Design review of the part built by this model. Coordinates are the model's own, in mm. A direction names the side the tool comes from. Round coordinates to 2 decimals unless told otherwise and drop trailing zeros. Order: outer loops, then holes, each group sorted by start corner. A loop starts at its lowest first (then second) coordinate and runs counter-clockwise, first axis right, second up. Notation, with made-up numbers: M 88,7.25 L 99,7.25 A34 cw 99,38.25 Z; hole C -32,-15 d7. An arc over 180 degrees is marked long. Write each question's results on one line, items separated by ' | '. Start each with the question number.
Item 1: Machinability: for faces 5 (the flat face through (-1, 50, 71)), 6 (the flat face through (150, 219, 573)), 7 (the flat face through (-4, 69, 140)), 8 (the flat face through (199, -150, 69)), which of the approach directions +Z, -Z, +X, -X, +Y, -Y give a long, thin tool a straight path to every point of the face, cutting with its end or side? Answer none if there is none.
Item 2: Wall thickness on line 1 (Z direction, x = 0, y = 358); line 2 (Z direction, x = -231.5, y = -60); line 3 (Y direction, x = -75.5, z = 316.5): over which ranges is each line inside the solid? List them lowest first. Write a range as [from, to].
Item 3: Take a section at C-C, the plane y = 336.5. Write out the cut boundary in (x, z), plus the area to 3 significant figures.
Item 4: The part is to be moulded in two halves that separate along Z. For faces 1 (the flat face through (4, 116, 0)), 2 (the flat face through (4, 390, 355)), 3 (the cylindrical face through (40.32, 339.3, 513.24)), 4 (the cylindrical face through (-3.298, 219.02, 300.036)), say which applies: +Z half, -Z half, draft (parallel to the pull), parting line (faces both ways), or undercut.
Item 5: Take a section at D-D, the plane z = 598. Write out the cut boundary in (x, y), plus the area to 3 significant figures.
Item 6: Clearance check with flat-ended pins moving along their axes: pin 1 (2 mm diameter, centred on x = 183.5, z = 331.5, fed in from -Y); pin 2 (3 mm diameter, centred on x = -94, z = 482, fed in from -Y). State where each tip first meets the part, or that it passes through.
Item 7: Take a section at B-B, the plane y = -69. Write out the cut boundary in (x, z).
Item 8: Take a section at A-A, the plane x = 0. Write out the cut boundary in (y, z).
```python
from build123d import *

# Parameters (mm, degrees)
F0_W     = 600
F0_H     = 300
F1_DEPTH = 140
F2_W     = 200
F2_H     = 200
F3_DEPTH = 140.001
F4_W     = 600
F4_H     = 700
F5_DEPTH = 240
F7_DEPTH = 140
F8_R     = 75
F9_DEPTH = 100.001


with BuildPart() as f1:
    # F0 (on Top) → F1 (new body)
    with BuildSketch(Plane.XY):
        Rectangle(F0_W, F0_H)
    extrude(amount=F1_DEPTH)

    # F2 (on face) → F3 (cut, through all)
    with BuildSketch(Plane.XY.offset(140)):
        with Locations((0, -50)):
            Rectangle(F2_W, F2_H)
    extrude(amount=-F3_DEPTH, mode=Mode.SUBTRACT)

    # F4 (on face) → F5 (join)
    with BuildSketch(Plane(origin=(0, 150, 0), x_dir=(-1, 0, 0), z_dir=(0, 1, 0))):
        with Locations((0, 350)):
            Rectangle(F4_W, F4_H)
    extrude(amount=F5_DEPTH)

    # F6 (on face) → F7 (cut)
    with BuildSketch(Plane.XZ.offset(-150)):
        with BuildLine():
            Line((150, 450), (150, 700))
            Line((150, 700), (-150, 700))
            Line((-150, 700), (-150, 450))
            ThreePointArc((-150, 450), (0, 300), (150, 450))
        make_face()
    extrude(amount=-F7_DEPTH, mode=Mode.SUBTRACT)

    # F8 (on face) → F9 (cut, through all)
    with BuildSketch(Plane.XZ.offset(-290)):
        with Locations((0, 450)):
            Circle(F8_R)
    extrude(amount=-F9_DEPTH, mode=Mode.SUBTRACT)


solid = f1.part
```
Results list:
1) face 5: +Z, -Z, -Y | face 6: +Z, -Y | face 7: +Z, +X, -X, -Y | face 8: +Z, -Z, +X, -X, -Y
2) line 1: [0, 375], [525, 700] | line 2: [0, 140] | line 3: [150, 390]
3) outline: M -300,0 L 300,0 L 300,700 L -300,700 Z; hole C 0,450 d150 | area: 402,000 mm²
4) face 1: -Z half | face 2: draft | face 3: undercut | face 4: +Z half
5) outline: M -300,150 L -150,150 L -150,290 L 150,290 L 150,150 L 300,150 L 300,390 L -300,390 Z | area: 102,000 mm²
6) pin 1: y = 150 | pin 2: y = 290
7) outline: M -300,0 L -100,0 L -100,140 L -300,140 Z; M 100,0 L 300,0 L 300,140 L 100,140 Z
8) outline: M 50,0 L 390,0 L 390,375 L 290,375 L 290,300 L 150,300 L 150,140 L 50,140 Z; M 290,525 L 390,525 L 390,700 L 290,700 Z
